Part model, mm, in its own coordinate system. Give positions to 0.01 mm unless a question says otherwise; leave off trailing zeros. Write each loop counter-clockwise with the first axis right and the second up, starting at its lowest first coordinate (ties: lowest second). Pieces come first, ordered by that corner, then holes. Notation, with made-up numbers: M 65,54 L 82,54 A27 ccw 82,83 Z; hole C 54.25,-18 d11. An arc over 180 degrees is marked long. Use a Markdown table: item, result.
```python
from build123d import *

# Parameters (mm, degrees)
BOSS_EXTRUDE1_DEPTH = 5
SKETCH2_W           = 5.7
SKETCH2_H           = 6.7
BOSS_EXTRUDE6_DEPTH = 24
SKETCH5_W           = 5
SKETCH5_H           = 6
BOSS_EXTRUDE7_DEPTH = 32
SKETCH4_R           = 1.4
BOSS_EXTRUDE4_DEPTH = 8


with BuildPart() as part:
    # Sketch1 → Boss-Extrude1 (new body)
    with BuildSketch(Plane.XY):
        Polygon((0, 6.7), (0, 8.05), (5.5, 8.05), (145.5, 8.05), (145.5, -42.1), (150.5, -42.1), (150.5, 8.05), (150.5, 12.9), (5.5, 12.9), (-4, 12.9), (-4, 0), (0, 0), (5.7, 0), (5.7, 6.7), align=None)
    extrude(amount=BOSS_EXTRUDE1_DEPTH)

    # Sketch2 → Boss-Extrude6 (add)
    with BuildSketch(Plane.XY.offset(5)):
        with Locations((2.85, 3.35)):
            Rectangle(SKETCH2_W, SKETCH2_H)
    extrude(amount=-BOSS_EXTRUDE6_DEPTH)

    # Sketch5 → Boss-Extrude7 (add)
    with BuildSketch(Plane(origin=(0, 0, 0), x_dir=(-1, 0, 0), z_dir=(0, 0, -1))):
        with Locations((-148, -39.1)):
            Rectangle(SKETCH5_W, SKETCH5_H)
    extrude(amount=BOSS_EXTRUDE7_DEPTH)

    # Sketch4 → Boss-Extrude4 (add)
    with BuildSketch(Plane.ZY.offset(-145.5)):
        with Locations(Location((-29, -39.1, 0), (0, 0, 180))):
            Circle(SKETCH4_R)
        with Locations(Location((2, -39.1, 0), (0, 0, 180))):
            Circle(SKETCH4_R)
    extrude(amount=BOSS_EXTRUDE4_DEPTH)


solid = part.part
```
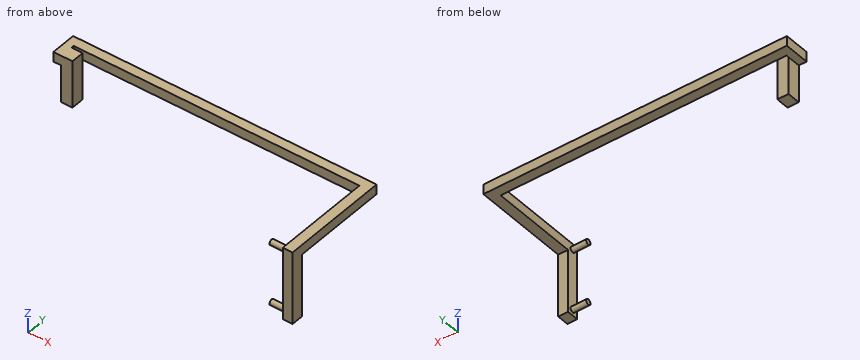
1. Cut at D-D, the plane x = 30.5. Give the cut face in (y, z), then the cut area to 4 significant figures.
Findings below:
| item | result |
|---|---|
| outline | M 8.05,0 L 12.9,0 L 12.9,5 L 8.05,5 Z |
| area | 24.25 mm2 |
2. Cut at A-A, the plane z = -9. Give the cut face in (x, y), then the cut area to 3 significant figures.
Findings below:
| item | result |
|---|---|
| outline | M 0,0 L 5.7,0 L 5.7,6.7 L 0,6.7 Z; M 145.5,-42.1 L 150.5,-42.1 L 150.5,-36.1 L 145.5,-36.1 Z |
| area | 68.2 mm2 |
3. Cut at C-C, the plane z = 2. Give the cut face in (x, y), then the cut area to 3 significant figures.
Findings below:
| item | result |
|---|---|
| outline | M -4,0 L 5.7,0 L 5.7,6.7 L 0,6.7 L 0,8.05 L 145.5,8.05 L 145.5,-37.7 L 137.5,-37.7 L 137.5,-40.5 L 145.5,-40.5 L 145.5,-42.1 L 150.5,-42.1 L 150.5,12.9 L -4,12.9 Z |
| area | 1,090 mm2 |
4. Drill centre lines: L1, parallel to Z at x = 125.5, y = 9; L2, parallel to Y at x = 3.5, z = -4; L3, parallel to X at y = -20.5, z = 3. Where is each one in solid material? Low to high.
Findings below:
| item | result |
|---|---|
| L1 | 0 to 5 |
| L2 | 0 to 6.7 |
| L3 | 145.5 to 150.5 |
5. Cut at B-B, the plane y = -39.1. Give the cut face in (x, z), then the cut area to 3 significant figures.
Findings below:
| item | result |
|---|---|
| outline | M 137.5,-30.4 L 145.5,-30.4 L 145.5,-32 L 150.5,-32 L 150.5,5 L 145.5,5 L 145.5,3.4 L 137.5,3.4 L 137.5,0.6 L 145.5,0.6 L 145.5,-27.6 L 137.5,-27.6 Z |
| area | 230 mm2 |
6. Drop flat-ended pins along their axis: P1, Ø4.5, axis at x = 4, y = 2.5, coming from the -Z side; P2, Ø7.5, axis at y = 2.5, z = -8, coming from the -X side; P3, Ø5.5, axis at y = 4, z = -12.5, coming from the +X side. Give the stop position or say it passes through.
Findings below:
| item | result |
|---|---|
| P1 | z = -19 |
| P2 | x = 0 |
| P3 | x = 5.7 |
